from build123d import *

# Parameters (mm, degrees)
SKETCH1_W           = 35
SKETCH1_H           = 100
BOSS_EXTRUDE1_DEPTH = 25
SKETCH2_W           = 19
SKETCH2_H           = 120
CUT_EXTRUDE1_DEPTH  = 25
FILLET2_RADIUS      = 12.5
FILLET2_LENGTH      = 8
FILLET3_RADIUS      = 12.5
FILLET3_LENGTH      = 8
SKETCH3_R           = 3.4
CUT_EXTRUDE2_DEPTH  = 70
SKETCH4_R           = 4.25
CUT_EXTRUDE3_DEPTH  = 45
SKETCH5_W           = 25
SKETCH5_H           = 30
CUT_EXTRUDE4_DEPTH  = 20
CHAMFER1_SIZE       = 2
FILLET4_R           = 5
SKETCH6_W           = 25
SKETCH6_H           = 10
CUT_EXTRUDE5_DEPTH  = 108.819293264
FILLET5_R           = 10
SKETCH7_W           = 19
SKETCH7_H           = 10
BOSS_EXTRUDE2_DEPTH = 5
FILLET6_R           = 4


with BuildPart() as part:
    # Sketch1 → Boss-Extrude1 (new body)
    with BuildSketch(Plane.XY):
        with Locations((17.5, 50)):
            Rectangle(SKETCH1_W, SKETCH1_H)
    extrude(amount=BOSS_EXTRUDE1_DEPTH)

    # Sketch2 → Cut-Extrude1 (cut)
    with BuildSketch(Plane.XY.offset(25)):
        with Locations((17.5, 100)):
            Rectangle(SKETCH2_W, SKETCH2_H)
    extrude(amount=-CUT_EXTRUDE1_DEPTH, mode=Mode.SUBTRACT)

    # Fillet2: full round fillet: the end face becomes a half cylinder, R = half its width
    fillet2_face = Plane((31, 100, 12.5), x_dir=(1, 0, 0), z_dir=(0, 1, 0))  # on the end face: x along it, z out of the body
    fillet2_slab = fillet2_face.offset(-FILLET2_RADIUS / 2) * Box(FILLET2_LENGTH, 2 * FILLET2_RADIUS, FILLET2_RADIUS, mode=Mode.PRIVATE)  # the body's end, R deep
    fillet2_round = Plane((31, 87.5, 12.5), x_dir=(0, 1, 0), z_dir=(1, 0, 0)) * Cylinder(FILLET2_RADIUS, FILLET2_LENGTH, mode=Mode.PRIVATE)  # its axis R under the face
    add(fillet2_slab - fillet2_round, mode=Mode.SUBTRACT)

    # Fillet3: full round fillet: the end face becomes a half cylinder, R = half its width
    fillet3_face = Plane((4, 100, 12.5), x_dir=(-1, 0, 0), z_dir=(0, 1, 0))  # on the end face: x along it, z out of the body
    fillet3_slab = fillet3_face.offset(-FILLET3_RADIUS / 2) * Box(FILLET3_LENGTH, 2 * FILLET3_RADIUS, FILLET3_RADIUS, mode=Mode.PRIVATE)  # the body's end, R deep
    fillet3_round = Plane((4, 87.5, 12.5), x_dir=(0, 1, 0), z_dir=(-1, 0, 0)) * Cylinder(FILLET3_RADIUS, FILLET3_LENGTH, mode=Mode.PRIVATE)  # its axis R under the face
    add(fillet3_slab - fillet3_round, mode=Mode.SUBTRACT)

    # Sketch3 → Cut-Extrude2 (cut)
    with BuildSketch(Plane.XZ):
        with Locations(Location((17.5, 12.5, 0), (0, 0, 270))):
            Circle(SKETCH3_R)
    extrude(amount=-CUT_EXTRUDE2_DEPTH, mode=Mode.SUBTRACT)

    # Sketch4 → Cut-Extrude3 (cut)
    with BuildSketch(Plane(origin=(35, 0, 0), x_dir=(0, 0, -1), z_dir=(1, 0, 0))):
        with Locations((-12.5, 87.5)):
            Circle(SKETCH4_R)
    extrude(amount=-CUT_EXTRUDE3_DEPTH, mode=Mode.SUBTRACT)

    # Sketch5 → Cut-Extrude4 (cut)
    with BuildSketch(Plane(origin=(0, 0, 0), x_dir=(-1, 0, 0), z_dir=(0, 0, -1))):
        with Locations((-17.5, 20)):
            Rectangle(SKETCH5_W, SKETCH5_H)
    extrude(amount=-CUT_EXTRUDE4_DEPTH, mode=Mode.SUBTRACT)

    # Chamfer1
    chamfer1_edges = [part.edges().sort_by_distance(p)[0] for p in [
        (17.5, 0, 0),
        (35, 0, 12.5),
        (0, 0, 12.5),
        (17.5, 0, 25),
    ]]
    chamfer(chamfer1_edges, length=CHAMFER1_SIZE)

    # Fillet4
    fillet4_edges = [part.edges().sort_by_distance(p)[0] for p in [
        (8, 40, 12.5),
        (27, 40, 12.5),
    ]]
    fillet(fillet4_edges, radius=FILLET4_R)

    # Sketch6 → Cut-Extrude5 (cut, through all)
    with BuildSketch(Plane(origin=(0, 0, 20), x_dir=(-1, 0, 0), z_dir=(0, 0, -1))):
        with Locations((-17.5, 30)):
            Rectangle(SKETCH6_W, SKETCH6_H)
        with Locations((-17.5, 10)):
            Rectangle(SKETCH6_W, SKETCH6_H)
    extrude(amount=-CUT_EXTRUDE5_DEPTH, mode=Mode.SUBTRACT)

    # Fillet5
    fillet5_edges = [part.edges().sort_by_distance(p)[0] for p in [
        (30, 15, 22.5),
        (30, 25, 22.5),
        (5, 25, 22.5),
        (5, 15, 22.5),
    ]]
    fillet(fillet5_edges, radius=FILLET5_R - 0.0001)  # a hair under: the kernel refuses the full size

    # Sketch7 → Boss-Extrude2 (add)
    with BuildSketch(Plane(origin=(0, 0, 0), x_dir=(-1, 0, 0), z_dir=(0, 0, -1))):
        with Locations((-17.5, 66.25)):
            Rectangle(SKETCH7_W, SKETCH7_H)
    extrude(amount=-BOSS_EXTRUDE2_DEPTH)

    # Fillet6
    fillet6_edges = [part.edges().sort_by_distance(p)[0] for p in [
        (8, 71.25, 2.5),
        (8, 61.25, 2.5),
        (27, 61.25, 2.5),
        (27, 71.25, 2.5),
    ]]
    fillet(fillet6_edges, radius=FILLET6_R)


solid = part.part
Input: part model. Units: mm. Frame: model coordinates. A direction names the side the tool comes from. Coordinates: 2 decimals unless noted, no trailing zeros. Loops run counter-clockwise (first coordinate to the right, second up) from the corner with the lowest first, then second, coordinate; pieces in that order, holes last. Notation, with made-up numbers: (79.5, 83) -> (85.5, 83) arc R24 cw to (85.5, 117) -> close; hole circle Ø8 at (-36, 35.5). An arc over 180 degrees is marked (long way). Write item = value, one per line. Start each with the question number.
Item 1: Cut plane D-D, the plane x = 31. Return loops of the section in (y, z), plus the area to 3 significant figures.
Item 2: First-contact query: P1, Ø7.5, axis at x = 14.5, z = 6.5, coming from the +Y side; P2, Ø10, axis at x = 13.5, y = 47.5, coming from the +Z side; P3, Ø4.5, axis at x = 17.5, z = 14, coming from the +Y side; P4, Ø10, axis at x = 26.5, z = 3, coming from the +Y side. Flat tips, straight axial feed; report the tip coordinate or a pass-through.
Item 3: Mould query, pull axis Y, two halves, no side actions, for faces 5 (the face through (0, 50, 12)), 6 (the face through (17, 1, 1)), 7 (the face through (8.01, 12.15, 22.54)). Classes: pulls with the +Y half, pulls with the -Y half, needs draft (parallel to the pull), parting line crosses it, or undercut.
Item 4: Reachability of faces 1 (the face through (8.01, 27.85, 22.54)), 2 (the face through (30, 20, 10)), 3 (the face through (25.859, 72.453, 2.535)), 4 (the face through (14.18, 37.47, 13.24)) from +Z, -Z, +X, -X, +Y, -Y: full face, straight path, thin tool, end or side. Return the list, or none.
Item 5: Cut plane C-C, the plane z = 12.5. Count the separate pieces of the cut face and the enclosed holes in it, plus the area to 3 significant figures.
Item 6: Material intervals for line 1 (Y direction, x = 18, z = 4.5); line 2 (X direction, y = 55, z = 13.25); line 3 (Y direction, x = 31.25, z = 12.5), sorted ascending.
Item 7: Cut plane A-A, the plane y = 49.5. Return loops of the section in (x, z), plus the area to 3 significant figures.
Item 8: Cut plane B-B, the plane x = 17.5. Return loops of the section in (y, z), plus the area to 3 significant figures.
Ans:
q1.outline = (0, 2) -> (2, 0) -> (87.5, 0) arc R12.5 ccw to (87.5, 25) -> (2, 25) -> (0, 23) -> close; hole circle Ø8.5 at (87.5, 12.5)
q1.area = 2,370 mm²
q2.P1 = 71.36
q2.P2 = through
q2.P3 = 40
q2.P4 = 99.15
q3.face_5 = needs draft
q3.face_6 = pulls with the -Y half
q3.face_7 = undercut
q4.face_1 = +Z, -Z
q4.face_2 = -Z
q4.face_3 = +Z, -Z, +Y
q4.face_4 = +Y, -Y
q5.separate_pieces = 4
q5.enclosed_holes = 0
q5.area = 1,410 mm²
q6.line_1 = 0 to 5, 35 to 40, 61.25 to 71.25
q6.line_2 = 0 to 8, 27 to 35
q6.line_3 = 0 to 83.25, 91.75 to 100
q7.outline = (0, 0) -> (8, 0) -> (8, 25) -> (0, 25) -> close; (27, 0) -> (35, 0) -> (35, 25) -> (27, 25) -> close
q7.area = 400 mm²
q8.outline = (0, 2) -> (2, 0) -> (5, 0) -> (5, 9.1) -> (0, 9.1) -> close; (0, 15.9) -> (5, 15.9) -> (5, 25) -> (2, 25) -> (0, 23) -> close; (15, 20) -> (25, 20) -> (25, 25) -> (15, 25) -> close; (35, 0) -> (40, 0) -> (40, 9.1) -> (35, 9.1) -> close; (35, 15.9) -> (40, 15.9) -> (40, 25) -> (35, 25) -> close; (61.25, 0) -> (71.25, 0) -> (71.25, 5) -> (61.25, 5) -> close
q8.area = 278 mm²
